Autodesk Inventor part; units mm, degrees
ref_plane "Work Plane1" through (-50.7483, 0, 0.135) normal (1, 0, 0) x (0, 0, -1)
ref_plane "YZ Plane" through (0, 0, 0) normal (1, 0, 0) x (0, 1, 0)
ref_plane "XZ Plane" through (0, 0, 0) normal (0, 1, 0) x (-1, 0, 0)
sketch "Sketch1" plane through (0, 0, 0) normal (0, 1, 0) x (-1, 0, 0)
  circle A0 centre (1.4663, 0.135) radius 40
  circle A1 centre (1.4663, 0.135) radius 60
  line L0 (55.7483, -8.5253) -> (-18.1747, -51.2048)
  line L1 (-33.1747, -42.5445) -> (-33.1747, 42.8145)
  line L2 (-18.1747, 51.4747) -> (55.7483, 8.7952)
  arc A2 (55.7483, -8.5253) -> (55.7483, 8.7952) centre (50.7483, 0.135) ccw
  arc A3 (-33.1747, -42.5445) -> (-18.1747, -51.2048) centre (-23.1747, -42.5445) ccw
  arc A4 (-18.1747, 51.4747) -> (-33.1747, 42.8145) centre (-23.1747, 42.8145) ccw
  point P0 (70.7483, 0.135)
  point P1 (-33.1747, -59.865)
  point P2 (-33.1747, 60.135)
  dimension "d2" = 120
  dimension "d3" = 10
extrude "Extrusion1" add sketch "Sketch1" along normal blind 12.7 contours A0 L0 L1 L2 | A0 L2 A2 L0 | A0 L1 A4 L2 | L0 A3 L1 A0
sketch "Sketch4" plane through (0, 0, 0) normal (0, -1, 0) x (1, 0, 0)
  line L0 (-55.7483, -8.5253) -> (18.1747, -51.2048)
  arc A0 (18.1747, -51.2048) -> (33.1747, -42.5445) centre (23.1747, -42.5445) ccw
  line L1 (33.1747, -42.5445) -> (33.1747, 42.8145)
  arc A1 (33.1747, 42.8145) -> (18.1747, 51.4747) centre (23.1747, 42.8145) ccw
  line L2 (18.1747, 51.4747) -> (-55.7483, 8.7952)
  arc A2 (-55.7483, 8.7952) -> (-55.7483, -8.5253) centre (-50.7483, 0.135) ccw
  point P0 (0, 0)
ref_plane "Work Plane1" through (-50.7483, 0, 0.135) normal (1, 0, 0) x (0, 0, -1)
sketch "Sketch6" plane through (0, 12.7, 0) normal (0, 1, 0) x (1, 0, 0)
  line L0 (18.1747, 51.2048) -> (-55.7483, 8.5253)
  arc A0 (-55.7483, 8.5253) -> (-55.7483, -8.7952) centre (-50.7483, -0.135) ccw
  line L1 (-55.7483, -8.7952) -> (18.1747, -51.4747)
  arc A1 (18.1747, -51.4747) -> (33.1747, -42.8145) centre (23.1747, -42.8145) ccw
  line L2 (33.1747, -42.8145) -> (33.1747, 42.5445)
  arc A2 (33.1747, 42.5445) -> (18.1747, 51.2048) centre (23.1747, 42.5445) ccw
  line L3 (23.1747, 42.5445) -> (23.1747, -42.8145) construction
  circle A3 centre (-50.7483, -0.135) radius 1.5 construction
  line L4 (-50.7483, -0.135) -> (23.1747, -0.135) construction
  line L5 (23.1747, 42.5445) -> (-50.7483, -0.135) construction
  line L6 (23.1747, -42.8145) -> (-13.7868, 21.2048) construction
  line L7 (-50.7483, -0.135) -> (23.1747, -42.8145) construction
  line L8 (23.1747, 42.5445) -> (-13.7868, -21.4747) construction
  circle A4 centre (-1.4663, -0.135) radius 17.5
  point P0 (0, 0)
  dimension "d38" = 35
hole "Hole1" at (-1.4663, 12.7, 0.135) direction (0, -1, 0) diameter 24.25 end through all
hole "Hole2" at (-50.7483, 12.7, 0.135) at (23.1747, 12.7, 42.8145) at (23.1747, 12.7, -42.5445) direction (0, -1, 0) diameter 5 end through all
thread "Thread1"
thread "Thread2"
thread "Thread3"
thicken "Thicken1" operation add thickness 0.2 both sides no extend neighbours yes toward (0, -1, 0) faces at (25.6399, 12.7, 0.6222)
thread "Thread4"
properties part number "Triangle_RK" material "white material"
Geometry: final body of the model. Coordinates: model frame, mm. Round coordinates to 2 decimals unless told otherwise and drop trailing zeros. Write each loop counter-clockwise with the first axis right and the second up, starting at its lowest first coordinate (ties: lowest second). Pieces come first, ordered by that corner, then holes. Notation, with made-up numbers: M -21.5,-6.75 L -6.5,-6.75 A26 ccw -6.5,25.25 Z; hole C 1,55 d9. An arc over 180 degrees is marked long. Write item = value, one per line.
Item 1: Material intervals for line 1 along Z through (x, y) = (6, 9); line 2 along Z through (x, y) = (-10.5, 10.25); line 3 along Z through (x, y) = (12.5, 8.5), sorted ascending. Write a range as [from, to].
Findings:
line_1 = [-44.18, -9.42], [9.69, 44.45]
line_2 = [-34.65, -7.95], [8.22, 34.92]
line_3 = [-47.93, 48.2]
Item 2: Pull-direction query (Z, two-part tool) for faces 1 (the face through (-3, 0, 13)), 2 (the face through (23.065, 6.162, 40.317)), 3 (the face through (28.3, 6.2, 51.4)); classes: pulls with the +Z half, pulls with the -Z half, needs draft (parallel to the pull), parting line crosses it, or undercut.
Findings:
face_1 = needs draft
face_2 = undercut
face_3 = pulls with the +Z half
Item 3: Section query B-B on x = 1. Return loops of the section in (y, z), then the cut area to 3 significant figures.
Findings:
outline = M 0,-41.29 L 12.5,-41.29 L 12.5,-11.74 L 0,-11.74 Z; M 0,12.01 L 12.5,12.01 L 12.5,41.56 L 0,41.56 Z
area = 739 mm^2
Item 4: Section query C-C on y = 9.75. State how many separate pieces and enclosed holes the cut face has, then the cut area to 3 significant figures.
Findings:
separate_pieces = 1
enclosed_holes = 4
area = 5,510 mm^2
Item 5: Section query D-D on x = -23. Return loops of the section in (y, z), then the cut area to 3 significant figures.
Findings:
outline = M 0,-27.43 L 12.5,-27.43 L 12.5,27.7 L 0,27.7 Z
area = 689 mm^2
Item 6: Section query A-A on z = -5. Return loops of the section in (x, y).
Findings:
outline = M -59.33,0 L -12.45,0 L -12.45,12.5 L -59.33,12.5 Z; M 9.52,0 L 33.17,0 L 33.17,12.5 L 9.52,12.5 Z
Item 7: Pin query (flat end, axial travel): P1, Ø1, axis at x = 10.5, y = 4, coming from the -Z side; P2, Ø1, axis at y = 6.5, z = 30.5, coming from the -X side; P3, Ø1.5, axis at y = 8, z = 23, coming from the -X side. Return the tip coordinate at first contact, or that it passes through.
Findings:
P1 = -47.06
P2 = -19.02
P3 = -32.44
